Check sheet for the drawn part. Datum: minimum x, y, z corner. Units: mm. Coordinates: 2 decimals unless noted, no trailing zeros. Order: outer loops, then holes, each group sorted by start corner. A loop starts at its lowest first (then second) coordinate and runs counter-clockwise, first axis right, second up. Notation, with made-up numbers: (-27.5, 13.25) - (-23.5, 13.25) arc R25 cw to (-23.5, 35.25) - close; hole circle Ø3 at (-31.5, 10.25). An arc over 180 degrees is marked (long way). Return JSON: item names as keys, results as strings. Group by question number.
Item 1: Section check A-A on z = 1.6. Enter the section's corners in (x, y).
Item 2: Section check D-D on x = 41. Enter the section's corners in (y, z).
Item 3: Section check B-B on y = 4. Enter the section's corners in (x, z), then the cut area to 3 significant figures.
Item 4: Scan lines: probe 1 along X at (y, z) = (4, 1.45); probe 2 along X at (y, z) = (5.5, 1.5); probe 3 along Y at (x, z) = (42.2, 1.3). Record each from-to range of solid material in increasing order.
Item 5: Gauge pin test, flat ends, axial feed: pin 1 (4 mm diameter, centred on x = 36, y = 5, fed in from -Z); pin 2 (3 mm diameter, centred on x = 21.2, y = 4, fed in from +Z). Record the tip position at first contact, or that the pin passes through.
Item 6: Section check C-C on x = 4.2. Enter the section's corners in (y, z).
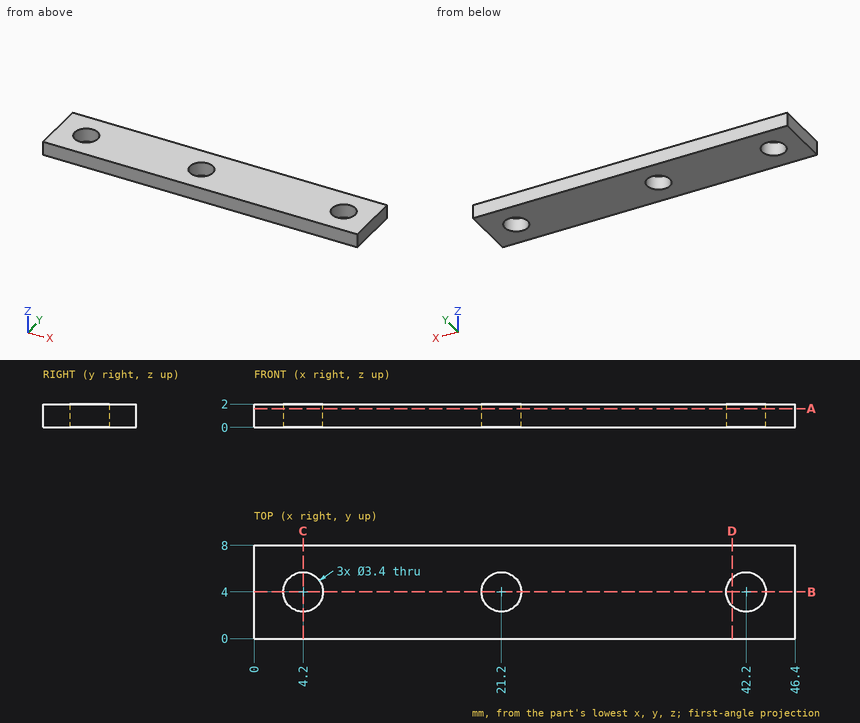
Computed:
{
 "1": {"outline": "(0, 0) - (46.4, 0) - (46.4, 8) - (0, 8) - close; hole circle Ø3.4 at (4.2, 4); hole circle Ø3.4 at (21.2, 4); hole circle Ø3.4 at (42.2, 4)"},
 "2": {"outline": "(0, 0) - (2.8, 0) - (2.8, 2) - (0, 2) - close; (5.2, 0) - (8, 0) - (8, 2) - (5.2, 2) - close"},
 "3": {"outline": "(0, 0) - (2.5, 0) - (2.5, 2) - (0, 2) - close; (5.9, 0) - (19.5, 0) - (19.5, 2) - (5.9, 2) - close; (22.9, 0) - (40.5, 0) - (40.5, 2) - (22.9, 2) - close; (43.9, 0) - (46.4, 0) - (46.4, 2) - (43.9, 2) - close", "area": "72.4 mm²"},
 "4": {"probe 1": "x = 0 to 2.5, 5.9 to 19.5, 22.9 to 40.5, 43.9 to 46.4", "probe 2": "x = 0 to 3.4, 5 to 20.4, 22 to 41.4, 43 to 46.4", "probe 3": "y = 0 to 2.3, 5.7 to 8"},
 "5": {"pin 1": "stops at z = 0", "pin 2": "passes through"},
 "6": {"outline": "(0, 0) - (2.3, 0) - (2.3, 2) - (0, 2) - close; (5.7, 0) - (8, 0) - (8, 2) - (5.7, 2) - close"}
}
